```python
from build123d import *

# Parameters (mm, degrees)
SKETCH1_R               = 3.96875
BOSS_EXTRUDE1_DEPTH     = 100
CUT_EXTRUDE2_DEPTH      = 101.157385914
CUT_EXTRUDE2_DEPTH_BACK = 101.157385914
SKETCH3_R               = 2
CUT_EXTRUDE3_DEPTH      = 101.157386022
CUT_EXTRUDE3_DEPTH_BACK = 101.157386022
SKETCH5_W               = 3
SKETCH5_H               = 4


with BuildPart() as part:
    # Sketch1 → Boss-Extrude1 (new body)
    with BuildSketch(Plane.XY):
        Circle(SKETCH1_R)
    extrude(amount=BOSS_EXTRUDE1_DEPTH)

    # Sketch3 → Cut-Extrude2 (cut, two sides: drawn at the far end of the back side and taken through both)
    with BuildSketch(Plane(origin=(0, 0, 0), x_dir=(1, 0, 0), z_dir=(0, 1, 0)).offset(-CUT_EXTRUDE2_DEPTH_BACK)):
        with Locations(Location((0, -5, 0), (0, 0, 270))):
            Circle(SKETCH3_R)
    extrude(amount=CUT_EXTRUDE2_DEPTH + CUT_EXTRUDE2_DEPTH_BACK, mode=Mode.SUBTRACT)

    # Sketch5 → Cut-Extrude3 (cut, two sides: drawn at the far end of the back side and taken through both)
    with BuildSketch(Plane(origin=(0, 0, 0), x_dir=(1, 0, 0), z_dir=(0, 1, 0)).offset(-CUT_EXTRUDE3_DEPTH_BACK)):
        with Locations((2.46875, -57)):
            Rectangle(SKETCH5_W, SKETCH5_H)
    extrude(amount=CUT_EXTRUDE3_DEPTH + CUT_EXTRUDE3_DEPTH_BACK, mode=Mode.SUBTRACT)


solid = part.part
```
The listing builds one solid part. Answer for the finished solid, in the listing's coordinates (mm). A direction names the side the tool comes from. Round coordinates to 2 decimals unless told otherwise and drop trailing zeros. Write each loop counter-clockwise with the first axis right and the second up, starting at its lowest first coordinate (ties: lowest second). Pieces come first, ordered by that corner, then holes. Notation, with made-up numbers: (-0.5, 26) -> (30.5, 26) arc R26 ccw to (30.5, 60) -> close; hole circle Ø6 at (-26.5, 69.5). An arc over 180 degrees is marked (long way). Write item = value, one per line.
1) Section B-B on x = 0 is taken. Write down the section's boundary in (y, z), plus the area to 3 significant figures.
Check values:
outline = (-3.97, 0) -> (3.97, 0) -> (3.97, 3) -> (-3.97, 3) -> close; (-3.97, 7) -> (3.97, 7) -> (3.97, 100) -> (-3.97, 100) -> close
area = 762 mm²
2) Section A-A on y = 0 is taken. Write down the section's boundary in (x, z).
Check values:
outline = (-3.97, 0) -> (3.97, 0) -> (3.97, 55) -> (0.97, 55) -> (0.97, 59) -> (3.97, 59) -> (3.97, 100) -> (-3.97, 100) -> close; hole circle Ø4 at (0, 5)
3) Section C-C on z = 49.5 is taken. Write down the section's boundary in (x, y).
Check values:
outline = circle Ø7.94 at (0, 0)
4) Section D-D on z = 5 is taken. Write down the section's boundary in (x, y).
Check values:
outline = (-2, -3.43) -> (-2, 3.43) arc R3.97 ccw to start; (2, -3.43) arc R3.97 ccw to (2, 3.43) -> close
5) For a pull along Z with two mould halves and no side action, classify faces 3 (the flat face through (0, 0, 100)), 4 (the flat face through (0, 0, 0)), 5 (the flat face through (0.969, 0, 57)) as released by +Z, released by -Z, zero draft, split by the parting line, or undercut.
Check values:
face_3 = released by +Z
face_4 = released by -Z
face_5 = undercut
6) Straight lines are drawn through the part: line 1 along Z through (x, y) = (2.5, 0.5); line 2 along Z through (x, y) = (0, 1); line 3 along Z through (x, y) = (1, -1.25). For each, find the intervals that lie inside material, in ascending order. Write a range as [from, to].
Check values:
line_1 = [0, 55], [59, 100]
line_2 = [0, 3], [7, 100]
line_3 = [0, 3.27], [6.73, 55], [59, 100]
7) Which of the six approach directions +Z, -Z, +X, -X, +Y, -Y give full straight-line access (tool end or side, diameter ignored) to faces 1 (the cylindrical face through (-0.517, 3.935, 49.3)), 2 (the flat face through (2, 0, 55))?
Check values:
face_1 = +Z, -Z
face_2 = +X, +Y, -Y
8) Given pin 1 (2 mm diameter, centred on x = -3, z = 34, fed in from -Y); pin 2 (1 mm diameter, centred on x = -3, z = 81.5, fed in from +Y), each flat-ended and moving along its own axis, determine where each tip first touches the part or whether it passes through.
Check values:
pin_1 = -3.43
pin_2 = 3.08
